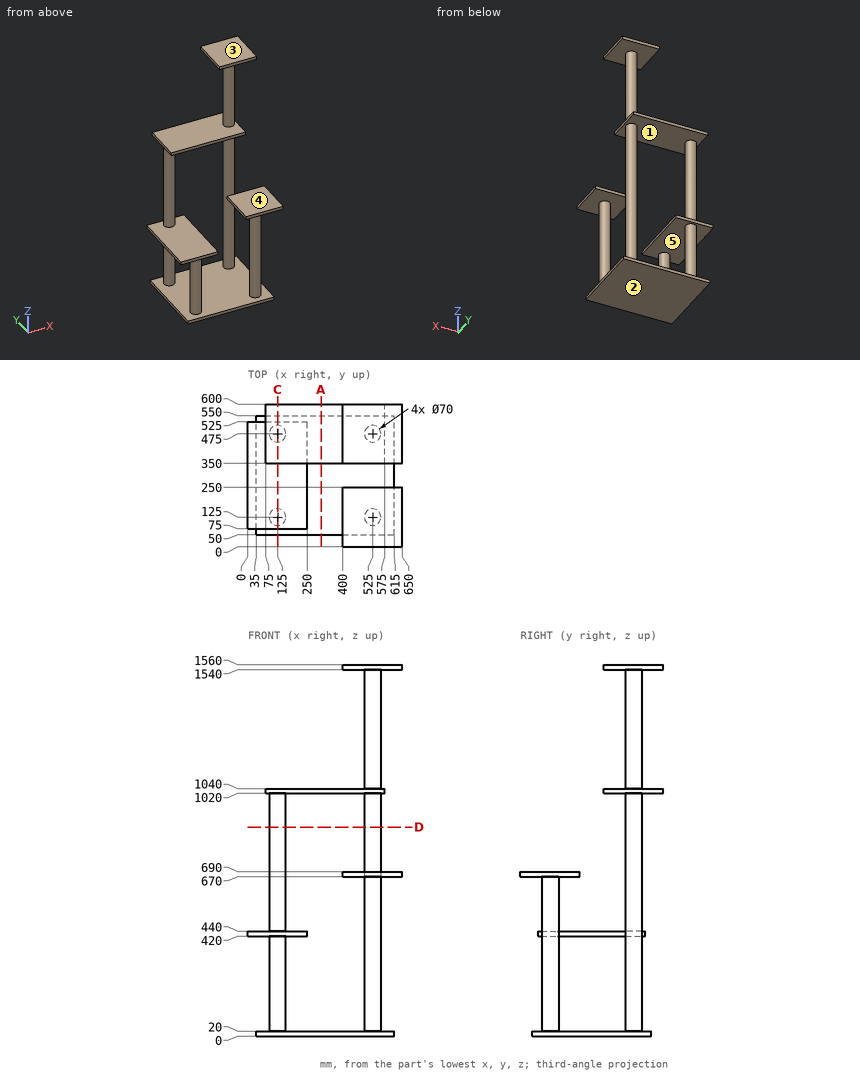
Could you check a few things on this drawing? It's one solid part, dimensions in mm from its lowest x, y, z. A direction names the side the tool comes from. Coordinates: 2 decimals unless noted, no trailing zeros. Order: outer loops, then holes, each group sorted by start corner. A loop starts at its lowest first (then second) coordinate and runs counter-clockwise, first axis right, second up. Notation, with made-up numbers: M 67,69 L 122,69 A16 cw 122,97 Z; hole C 73,-8.75 d6. An arc over 180 degrees is marked long. Answer as CSV lines item,"result".
(1) I'm going to push flat-ended pins straight in: pin 1 (6 mm diameter, centred on y = 505.5, z = 1028.5, fed in from -X); pin 2 (1.5 mm diameter, centred on x = 142.5, z = 610, fed in from -Y); pin 3 (4 mm diameter, centred on y = 446, z = 1086, fed in from +X); pin 4 (10 mm diameter, centred on y = 433, z = 777, fed in from +X). Where does each tip first touch, or does it pass through?
Geometry check:
pin 1,"x = 75"
pin 2,"y = 444.27"
pin 3,"x = 547.27"
pin 4,"through"
(2) If we mould it in two halves opening along X, with no side actions, what happens to the marked faces 1 and 2? For each: released by +X, released by -X, zero draft, split by the parting line, or undercut.
Geometry check:
face 1,"undercut"
face 2,"zero draft"
(3) Suppose I cut it at D-D on z = 878. Please give me the cut outline in (x, y).
Geometry check:
outline,"C 125,475 d70; C 525,475 d70"
(4) On a 3-axis mill with a long thin cutter (end or side, diameter ignored), from which of +Z, -Z, +X, -X, +Y, -Y can I reach the whole of each face in a straight line? I mean the marked faces 3, 4 and 5. Say none if no direction works.
Geometry check:
face 3,"+Z, +X, -X, +Y, -Y"
face 4,"+Z, +X, -X, -Y"
face 5,"none"
(5) Suppose I cut it at A-A on x = 308. Please give me the cut outline in (y, z).
Geometry check:
outline,"M 50,0 L 550,0 L 550,20 L 50,20 Z; M 350,1020 L 600,1020 L 600,1040 L 350,1040 Z"
(6) Please list where these lines run through material, in increasing order: L1, parallel to Z at x = 558, y = 391.5; L2, parallel to Z at x = 601.5, y = 388; L3, parallel to Z at x = 242, y = 125.
Geometry check:
L1,"0 to 20, 1020 to 1040, 1540 to 1560"
L2,"0 to 20, 1540 to 1560"
L3,"0 to 20, 420 to 440"
(7) Suppose I cut it at C-C on x = 125. Please give me the cut outline in (y, z).
Geometry check:
outline,"M 50,0 L 550,0 L 550,20 L 510,20 L 510,420 L 525,420 L 525,440 L 510,440 L 510,1020 L 600,1020 L 600,1040 L 350,1040 L 350,1020 L 440,1020 L 440,440 L 75,440 L 75,420 L 90,420 L 90,20 L 50,20 Z; hole M 160,20 L 440,20 L 440,420 L 160,420 Z"
